Autodesk Inventor part; units mm, degrees
ref_plane "YZ Plane" through (0, 0, 0) normal (1, 0, 0) x (0, 1, 0)
ref_plane "XZ Plane" through (0, 0, 0) normal (0, 1, 0) x (-1, 0, 0)
ref_plane "XY Plane" through (0, 0, 0) normal (0, 0, 1) x (1, 0, 0)
sketch "スケッチ1" plane through (0, 0, 0) normal (0, 0, 1) x (1, 0, 0)
  line L0 (122.5, -197.5) -> (-122.5, -197.5)
  line L1 (-122.5, -197.5) -> (-122.5, 197.5)
  line L2 (-122.5, 197.5) -> (122.5, 197.5)
  line L3 (122.5, 197.5) -> (122.5, -197.5)
  line L4 (122.5, -197.5) -> (-122.5, 197.5) construction
  line L5 (-122.5, -197.5) -> (122.5, 197.5) construction
  point P0 (0, 0)
  dimension "d0" = 245
  dimension "d1" = 395
extrude "押し出し1" add sketch "スケッチ1" along normal blind 15
sketch "スケッチ2" plane through (0, 0, 15) normal (0, 0, 1) x (1, 0, 0)
  line L0 (-122.5, 197.5) -> (-122.5, -197.5)
  line L1 (122.5, 197.5) -> (-122.5, 197.5)
  point P0 (0, 0)
  point P1 (-32.5, 37.5)
  point P2 (-32.5, -37.5)
  dimension "d4" = 90
  dimension "d5" = 75
  dimension "d6" = 160
hole "穴1" at (-32.5, 37.5, 15) at (-32.5, -37.5, 15) direction (0, 0, -1) diameter 4.134 depth 6 tip angle 118
sketch "スケッチ3" plane through (0, 0, 0) normal (0, 0, -1) x (-1, 0, 0)
  line L0 (122.5, -197.5) -> (-122.5, -197.5)
  line L1 (122.5, 197.5) -> (122.5, -197.5)
  line L2 (-122.5, 197.5) -> (122.5, 197.5)
  line L3 (-122.5, -197.5) -> (-122.5, 197.5)
  line L4 (102.5, 192.5) -> (-117.5, 192.5)
  line L5 (-117.5, 192.5) -> (-117.5, -192.5)
  line L6 (-117.5, -192.5) -> (102.5, -192.5)
  line L7 (102.5, -192.5) -> (102.5, 192.5)
  point P0 (0, 0)
  dimension "d14" = 5
  dimension "d15" = 5
  dimension "d16" = 5
  dimension "d17" = 20
extrude "押し出し2" cut sketch "スケッチ3" against normal blind 0.5 contours L7 L6 L5 L4
fillet "フィレット1" radius 5 4 edges at (122.5, -197.5, 7.5) (-122.5, -197.5, 7.5) (122.5, 197.5, 7.5) (-122.5, 197.5, 7.5)
properties part number "Display"
CAD build for the part. Positions are in the model's coordinates, mm. Round coordinates to 2 decimals unless told otherwise and drop trailing zeros. Loops run counter-clockwise (first coordinate to the right, second up) from the corner with the lowest first, then second, coordinate; pieces in that order, holes last.
(1) Drop flat-ended pins along their axis: pin 1 (2.5 mm diameter, centred on x = -32.5, y = -37.5, fed in from +Z); pin 2 (1.5 mm diameter, centred on x = 3.5, y = -110.5, fed in from -Z); pin 3 (3.5 mm diameter, centred on x = -32.5, y = 37.5, fed in from +Z). Give the stop position or say it passes through.
(2) Cut at A-A (x = 53.5). Give the cut face in (y, z).
(3) Two-plate mould, pull along X, no slides. Class faces 1 (the flat face through (122.5, 3, 7)), 2 (the flat face through (-2, 3, 15)), 3 (the flat face through (9, 3, 0.5)): +X half, -X half, draft (parallel to the pull), parting line (faces both ways), or undercut.
(4) Wall check: line 1 along Y through (x, z) = (-32.5, 10.45); line 2 along X through (y, z) = (-37.5, 12); line 3 along Z through (x, y) = (38.5, -92). Give the ranges that are in metal, low to high.
(5) Cut at B-B (y = -172.5). Give the cut face in (x, z), plus the area to 4 significant figures.
Findings below:
1. pin 1: stops at z = 8.51
1. pin 2: stops at z = 0.5
1. pin 3: stops at z = 8.81
2. outline: (-197.5, 0) - (-192.5, 0) - (-192.5, 0.5) - (192.5, 0.5) - (192.5, 0) - (197.5, 0) - (197.5, 15) - (-197.5, 15) - close
3. face 1: +X half
3. face 2: draft
3. face 3: undercut
4. line 1: y = -197.5 to -39.57, -35.43 to 35.43, 39.57 to 197.5
4. line 2: x = -122.5 to -34.57, -30.43 to 122.5
4. line 3: z = 0.5 to 15
5. outline: (-122.5, 0) - (-102.5, 0) - (-102.5, 0.5) - (117.5, 0.5) - (117.5, 0) - (122.5, 0) - (122.5, 15) - (-122.5, 15) - close
5. area: 3,565 mm2
